Autodesk Inventor part; units mm, degrees
ref_plane "YZ Plane" through (0, 0, 0) normal (1, 0, 0) x (0, 1, 0)
ref_plane "XZ Plane" through (0, 0, 0) normal (0, 1, 0) x (-1, 0, 0)
ref_plane "XY Plane" through (0, 0, 0) normal (0, 0, 1) x (1, 0, 0)
sketch "Sketch2" plane through (0, 0, 0) normal (0, 1, 0) x (-1, 0, 0)
  circle A0 centre (25.2851, 7.8895) radius 2.95
  circle A1 centre (25.2851, 7.8895) radius 4.75
  line L0 (25.2851, 3.1395) -> (33.2851, 3.1395)
  line L1 (25.2851, 12.6395) -> (33.2851, 12.6395)
  line L2 (33.2851, 3.1395) -> (33.2851, -4.0935)
  line L3 (33.2851, -4.0935) -> (43.6851, -4.0935)
  arc A2 (43.6851, -4.0935) -> (49.4162, 4.6499) centre (43.6851, 2.1565) ccw
  line L4 (49.4162, 4.6499) -> (44.7437, 15.3895)
  line L5 (44.7437, 15.3895) -> (33.2851, 15.3895)
  line L6 (33.2851, 15.3895) -> (33.2851, 12.6395)
  point P0 (0, 0)
  dimension "d0" = 5.9
  dimension "d1" = 9.5
  dimension "d2" = 8
  dimension "d4" = 10.4
  dimension "d21" = 11.983
  dimension "d22" = 6.25
extrude "Extrusion1" add sketch "Sketch2" along normal mid plane 5
sketch "Sketch4" plane through (0, 2.5, 0) normal (0, 1, 0) x (1, 0, 0)
  line L0 (-33.2851, -3.1395) -> (-33.2851, 4.0935)
  line L1 (-44.7437, -15.3895) -> (-33.2851, -15.3895)
  line L2 (-33.2851, 4.0935) -> (-37.2851, 4.0935)
  line L3 (-37.2851, 4.0935) -> (-37.2851, -15.3895)
  line L4 (-37.2851, -15.3895) -> (-33.2851, -15.3895)
  line L5 (-33.2851, -15.3895) -> (-33.2851, 4.0935)
  point P0 (0, 0)
  dimension "d8" = 4
extrude "Extrusion2" add sketch "Sketch4" along normal blind 9.25
sketch "Sketch5" plane through (0, 11.75, 0) normal (0, 1, 0) x (1, 0, 0)
  line L0 (-37.2851, -15.3895) -> (-37.2851, 4.0935)
  line L1 (-37.2851, 4.0935) -> (-43.6851, 4.0935)
  arc A0 (-43.6851, 4.0935) -> (-49.4162, -4.6499) centre (-43.6851, -2.1565) ccw
  line L2 (-49.4162, -4.6499) -> (-44.7437, -15.3895)
  line L3 (-44.7437, -15.3895) -> (-37.2851, -15.3895)
  point P0 (0, 0)
extrude "Extrusion3" add sketch "Sketch5" against normal blind 4.5
ref_plane "Work Plane1" through (0, 0, 0) normal (0, 1, 0) x (1, 0, 0)
mirror "Mirror1" about plane through (0, 0, 0) normal (0, 1, 0) of "Extrusion2", "Extrusion3"
sketch "Sketch6" plane through (-44.7437, -7.25, 15.3895) normal (0, 1, 0) x (1, 0, 0)
  point P0 (44.7437, 15.3895)
chamfer "Chamfer1" distance 2 angle 45 1 edges at (-33.2851, 0, 12.6395)
fillet "Fillet2" radius 4 2 edges at (-33.2851, 11.75, 5.648) (-33.2851, -11.75, 5.648)
sketch "Sketch7" plane through (-44.7437, -7.25, 15.3895) normal (0, 1, 0) x (1, 0, 0)
  arc A0 (1.0586, 19.483) -> (-4.6725, 10.7396) centre (1.0586, 13.233) ccw
  circle A1 centre (0.0586, 12.733) radius 1.75
  circle A2 centre (0.0586, 12.733) radius 6.75
  line L0 (1.0586, 19.483) -> (7.4586, 19.483)
  line L1 (1.0586, 19.483) -> (-38.3116, 19.483) construction
  point P0 (44.7437, 15.3895)
  dimension "d18" = 3.5
  dimension "d24" = 13.5
  dimension "d25" = 1
  dimension "d26" = 0.5
extrude "Extrusion4" add sketch "Sketch7" along normal up to surface (14.5 mm away) contours A1
sketch "Sketch8" plane through (0, 11.75, 0) normal (0, 1, 0) x (1, 0, 0)
  line L0 (-54.2603, -7.4065) -> (-37.2851, -7.4065)
  line L1 (-37.2851, -7.4065) -> (-37.2851, -23.5954)
  line L2 (-37.2851, 4.0935) -> (-37.2851, -15.3895)
  line L3 (-37.2851, 4.0935) -> (-43.6851, 4.0935)
  arc A0 (-43.6851, 4.0935) -> (-49.4162, -4.6499) centre (-43.6851, -2.1565) ccw
  line L4 (-49.4162, -4.6499) -> (-44.7437, -15.3895)
  line L5 (-44.7437, -15.3895) -> (-37.2851, -15.3895)
  point P0 (0, 0)
  point P1 (-48.2169, -7.4065)
  dimension "d28" = 11.5
extrude "Extrusion5" cut sketch "Sketch8" against normal up to surface (4.5 mm away) contours L0 L1 L5 L4
mirror "Mirror2" about plane through (0, 0, 0) normal (0, 1, 0) of "Extrusion5"
fillet "Fillet3" radius 3 2 edges at (-48.2169, 9.5, 7.4065) (-37.2851, 9.5, 7.4065)
fillet "Fillet4" radius 3 2 edges at (-48.2169, -9.5, 7.4065) (-37.2851, -9.5, 7.4065)
fillet "Fillet5" radius 5 1 edges at (-44.7437, 0, 15.3895)
fillet "Fillet6" radius 1 2 edges at (-37.2851, 7.125, 15.3895) (-37.2851, -7.125, 15.3895)
chamfer "Chamfer2" distance 7.23 angle 45 1 edges at (-33.2851, 0, 3.1395)
properties part number "hIP"
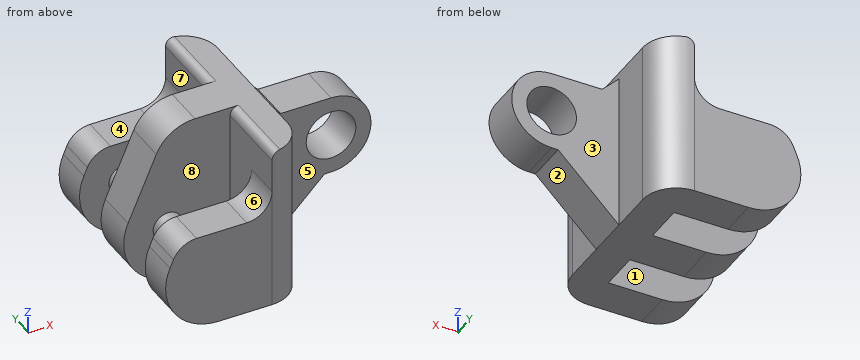
CAD build for the part. Positions are in the model's coordinates, mm. Face numbers are marked on the shaded views. A direction names the side the tool comes from. Give positions to 0.01 mm unless a question says otherwise; leave off trailing zeros. Order: outer loops, then holes, each group sorted by start corner. A loop starts at its lowest first (then second) coordinate and runs counter-clockwise, first axis right, second up.
(1) Drill centre lines: L1, parallel to Y at x = -48, z = -1; L2, parallel to X at y = 5.25, z = 5.75; L3, parallel to Z at x = -25.25, y = -0.75. Where is each one in solid material? Low to high.
(2) Saw through at C-C, the plane z = 1.5. Give the cut face in (x, y).
(3) Saw through at D-D, the plane y = 8.25. Give the cut face in (x, z), then the cut area to 3 significant figures.
(4) Saw through at B-B, the plane y = -3. Give the cut face in (x, z).
(5) Flat gauge pins, fed straight in: pin 1 (4 mm diameter, centred on x = -29.5, z = 1.5, fed in from -Y); pin 2 (5 mm diameter, centred on x = -44.5, y = 9.5, fed in from +Z); pin 3 (4 mm diameter, centred on x = -29.5, y = -1, fed in from +Z). Where does each tip first touch, or does it go through?
(6) Tool access for the marked faces 4, 5, 6, 7 and 8: list every direction of +Z, -Z, +X, -X, +Y, -Y with a clear straight run to the whole face (end or side of a thin tool).
(7) Mould opens along X. For the marked faces 1, 2 and 3 say: released by +X, released by -X, zero draft, split by the parting line, or undercut.
(8) Saw through at A-A, the plane x = -47.5. Give the cut face in (y, z).
Results found:
1. L1: y = -11.75 to -7.25, -2.5 to 2.5, 7.25 to 11.75
1. L2: x = -37.29 to -33.29
1. L3: z = 3.14 to 4.94, 10.84 to 12.64
2. outline: (-49.9, -11.75) - (-37.29, -11.75) arc R4 ccw to (-33.29, -7.75) - (-33.29, -2.5) - (-27.69, -2.5) - (-27.69, 2.5) - (-33.29, 2.5) - (-33.29, 7.75) arc R4 ccw to (-37.29, 11.75) - (-49.9, 11.75) - (-49.9, 7.25) - (-46, 7.25) - (-46, 2.5) - (-49.9, 2.5) - (-49.9, -2.5) - (-46, -2.5) - (-46, -7.25) - (-49.9, -7.25) - close; hole (-43.37, -7.25) - (-37.29, -7.25) - (-37.29, -2.5) - (-43.37, -2.5) - close; hole (-43.37, 2.5) - (-37.29, 2.5) - (-37.29, 7.25) - (-43.37, 7.25) - close
3. outline: (-49.42, 4.65) arc R6.25 ccw to (-43.69, -4.09) - (-33.32, -4.09) - (-33.32, 15.39) - (-36.29, 15.39) arc R1 ccw to (-37.29, 14.39) - (-37.29, 10.41) arc R3 cw to (-40.29, 7.41) - (-46.25, 7.41) arc R3 ccw to (-49, 5.6) - close
3. area: 212 mm2
4. outline: circle Ø3.5 at (-44.69, 2.66); (-37.29, -4.09) - (-33.29, -4.09) - (-33.29, 15.39) - (-36.29, 15.39) arc R1 ccw to (-37.29, 14.39) - close
5. pin 1: stops at y = -2.5
5. pin 2: stops at z = 7.41
5. pin 3: stops at z = 12.85
6. face 4: +Z, -X, +Y
6. face 5: +Z, -Z, +X, -Y
6. face 6: +Z, -X, -Y
6. face 7: +Z
6. face 8: none
7. face 1: undercut
7. face 2: released by +X
7. face 3: zero draft
8. outline: (-11.75, -2.79) - (-7.25, -2.79) - (-7.25, 7.13) - (-11.75, 7.13) - close; (-2.5, -2.79) - (2.5, -2.79) - (2.5, 9.05) - (-2.5, 9.05) - close; (7.25, -2.79) - (11.75, -2.79) - (11.75, 7.13) - (7.25, 7.13) - close
